For this review, take the finished solid that the model builds, in its own axes (mm). Face numbers are marked on the shaded views. A direction names the side the tool comes from. Coordinates: 2 decimals unless noted, no trailing zeros. Write each loop counter-clockwise with the first axis right and the second up, starting at its lowest first coordinate (ties: lowest second). Pieces come first, ordered by that corner, then holes.
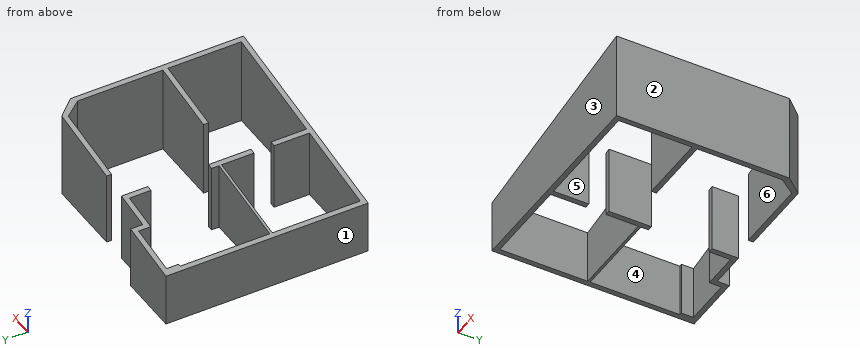
```python
from build123d import *

# Parameters (mm, degrees)
F1_DEPTH = 35
F3_DEPTH = 90


with BuildPart() as f1:
    # F0 (on Top) → F1 (new body)
    with BuildSketch(Plane.XY):
        Polygon((-50.260506, 1.061057), (-50.260506, 36.561057), (-49.260506, 36.561057), (-49.260506, 41.361057), (-30.060506, 41.361057), (-30.060506, 36.561057), (-15.460506, 36.561057), (-15.460506, 28.061057), (-13.460506, 28.061057), (-13.460506, 38.561057), (-28.060506, 38.561057), (-28.060506, 43.361057), (-50.260506, 43.361057), (-52.260506, 43.361057), (-52.260506, -36.738943), (-13.460506, -36.738943), (33.239494, -36.738943), (33.239494, 31.816978), (27.439494, 38.561057), (-3.260506, 38.561057), (-3.260506, 36.561057), (26.439494, 36.561057), (31.239494, 30.135054), (31.239494, -3.638943), (3.339494, -3.638943), (3.339494, -5.638943), (31.239494, -5.638943), (31.239494, -34.738943), (-13.460506, -34.738943), (-13.460506, -20.738943), (-15.460506, -20.738943), (-15.460506, -34.738943), (-50.260506, -34.738943), (-50.260506, 0.061057), (-15.460506, 0.061057), (-15.460506, -12.738943), (-13.460506, -12.738943), (-13.460506, 4.061057), (-15.460506, 4.061057), (-15.487555, 1.061057), align=None)
    extrude(amount=F1_DEPTH)

    # F2 (on face) → F3 (cut)
    with BuildSketch(Plane.XZ.offset(36.738943)):
        Polygon((-52.260506, 61.379157), (-52.260506, 21), (33.239494, 35), (27.843312, 67.955256), align=None)
    extrude(amount=-F3_DEPTH, mode=Mode.SUBTRACT)


solid = f1.part
```
Q1. Clearance check with flat-ended pins moving along their axes: pin 1 Ø4.5 at (x, z) = (-19.5, 7.5) entering from +Y; pin 2 Ø11.5 at (y, z) = (34, 13) entering from +X; pin 3 Ø4 at (y, z) = (41.5, 17.5) entering from +X; pin 4 Ø6 at (x, y) = (-35, -1.5) entering from +Z. State where each tip first meets the part, or that it passes through.
Ans:
pin 1: stops at y = 38.56
pin 2: stops at x = 33.24
pin 3: stops at x = -28.06
pin 4: stops at z = 24.25
Q2. Add section D-D (z = 23). Give the number of separate pieces and of enclosed holes in the cut face, then the cut area to 3 significant figures.
Ans:
separate pieces: 3
enclosed holes: 0
area: 580 mm2
Q3. Add section B-B (x = 14.5). State the section outline as (y, z) points.
Ans:
outline: (-36.74, 0) - (-34.74, 0) - (-34.74, 31.93) - (-36.74, 31.93) - close; (-5.64, 0) - (-3.64, 0) - (-3.64, 31.93) - (-5.64, 31.93) - close; (36.56, 0) - (38.56, 0) - (38.56, 31.93) - (36.56, 31.93) - close
Q4. For probe 1 along Y at (x, z) = (26, 25); probe 2 along Y at (x, z) = (-44, 20); probe 3 along X at (y, z) = (-26.5, 16.5), list the stretches that pass through material, from the lowest coordinate up.
Ans:
probe 1: y = -36.74 to -34.74, -5.64 to -3.64, 36.56 to 38.56
probe 2: y = -36.74 to -34.74, 0.06 to 1.06, 41.36 to 43.36
probe 3: x = -52.26 to -50.26, -15.46 to -13.46, 31.24 to 33.24
Q5. Add section C-C (y = 18.5). State the section outline as (x, z) points.
Ans:
outline: (-52.26, 0) - (-50.26, 0) - (-50.26, 21.33) - (-52.26, 21) - close; (31.24, 0) - (33.24, 0) - (33.24, 35) - (31.24, 34.67) - close
Q6. Tool access review of the marked faces 5 and 6: name each direction out of +Z, -Z, +X, -X, +Y, -Y from which nothing blocks a thin tool from reaching the whole face with its end or side.
Ans:
face 5: +Z, -Z, +Y
face 6: +Z, -Z
Q7. Add section A-A (y = -32). State the section outline as (x, z) points.
Ans:
outline: (-52.26, 0) - (-50.26, 0) - (-50.26, 21.33) - (-52.26, 21) - close; (-15.46, 0) - (-13.46, 0) - (-13.46, 27.35) - (-15.46, 27.03) - close; (31.24, 0) - (33.24, 0) - (33.24, 35) - (31.24, 34.67) - close
Q8. Draft analysis for pull direction X (two halves, no side actions). For the marked faces 1, 2, 3 and 4, state which applies: +X half, -X half, draft (parallel to the pull), parting line (faces both ways), or undercut.
Ans:
face 1: -X half
face 2: +X half
face 3: draft
face 4: undercut
